```python
from build123d import *

# Parameters (mm, degrees)
SKETCH1_W           = 90
SKETCH1_H           = 90
BOSS_EXTRUDE1_DEPTH = 11.45
SKETCH2_R           = 41
BOSS_EXTRUDE2_DEPTH = 52.45
SKETCH3_R           = 29.05
BOSS_EXTRUDE3_DEPTH = 19
SKETCH4_R           = 32.5
BOSS_EXTRUDE4_DEPTH = 12
SKETCH5_R           = 28
BOSS_EXTRUDE5_DEPTH = 12
SKETCH6_R           = 2.5
CUT_EXTRUDE1_DEPTH  = 115.720105038


with BuildPart() as part:
    # Sketch1 → Boss-Extrude1 (new body)
    with BuildSketch(Plane(origin=(0, 0, 0), x_dir=(1, 0, 0), z_dir=(0, 1, 0))):
        Rectangle(SKETCH1_W, SKETCH1_H)
    extrude(amount=BOSS_EXTRUDE1_DEPTH)

    # Sketch2 → Boss-Extrude2 (add)
    with BuildSketch(Plane(origin=(0, 11.45, 0), x_dir=(1, 0, 0), z_dir=(0, 1, 0))):
        with Locations(Location((0, 0, 0), (0, 0, 270))):
            Circle(SKETCH2_R)
    extrude(amount=BOSS_EXTRUDE2_DEPTH)

    # Sketch3 → Boss-Extrude3 (add)
    with BuildSketch(Plane(origin=(0, 63.9, 0), x_dir=(1, 0, 0), z_dir=(0, 1, 0))):
        with Locations(Location((0, 0, 0), (0, 0, 270))):
            Circle(SKETCH3_R)
    extrude(amount=BOSS_EXTRUDE3_DEPTH)

    # Sketch4 → Boss-Extrude4 (add)
    with BuildSketch(Plane(origin=(0, 82.9, 0), x_dir=(1, 0, 0), z_dir=(0, 1, 0))):
        with Locations(Location((0, 0, 0), (0, 0, 270))):
            Circle(SKETCH4_R)
    extrude(amount=BOSS_EXTRUDE4_DEPTH)

    # Sketch5 → Boss-Extrude5 (add)
    with BuildSketch(Plane(origin=(0, 94.9, 0), x_dir=(1, 0, 0), z_dir=(0, 1, 0))):
        with Locations(Location((0, 0, 0), (0, 0, 270))):
            Circle(SKETCH5_R)
    extrude(amount=BOSS_EXTRUDE5_DEPTH)

    # Sketch6 → Cut-Extrude1 (cut, through all)
    with BuildSketch(Plane(origin=(0, 11.45, 0), x_dir=(1, 0, 0), z_dir=(0, 1, 0))):
        with Locations(Location((-35, 36.75, 0), (0, 0, 270))):
            Circle(SKETCH6_R)
        with Locations(Location((35, 36.75, 0), (0, 0, 270))):
            Circle(SKETCH6_R)
        with Locations(Location((35, -36.75, 0), (0, 0, 270))):
            Circle(SKETCH6_R)
        with Locations(Location((-35, -36.75, 0), (0, 0, 270))):
            Circle(SKETCH6_R)
    extrude(amount=-CUT_EXTRUDE1_DEPTH, mode=Mode.SUBTRACT)


solid = part.part
```
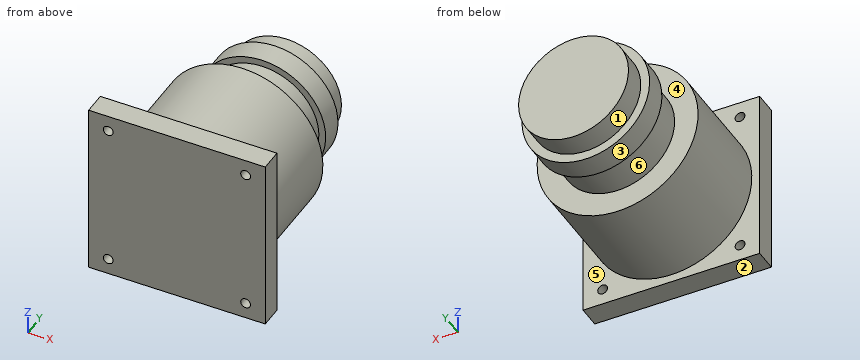
CAD build for the part. Positions are in the model's coordinates, mm. Face numbers are marked on the shaded views. A direction names the side the tool comes from. Round coordinates to 2 decimals unless told otherwise and drop trailing zeros. Write each loop counter-clockwise with the first axis right and the second up, starting at its lowest first coordinate (ties: lowest second). Pieces come first, ordered by that corner, then holes.
Item 1: Band-saw the part on B-B on x = 35. Write the cut outline in (y, z).
Filled in:
outline: (0, -45) - (11.45, -45) - (11.45, -39.25) - (0, -39.25) - close; (0, -34.25) - (11.45, -34.25) - (11.45, -21.35) - (63.9, -21.35) - (63.9, 21.35) - (11.45, 21.35) - (11.45, 34.25) - (0, 34.25) - close; (0, 39.25) - (11.45, 39.25) - (11.45, 45) - (0, 45) - close
Item 2: Drop flat-ended pins along their axis: pin 1 Ø1.5 at (y, z) = (53.5, 36) entering from -X; pin 2 Ø6.5 at (x, z) = (-35, -36.75) entering from +Y; pin 3 Ø1 at (x, y) = (-21, 53) entering from -Z; pin 4 Ø4 at (x, z) = (35, -36.75) entering from +Y. Give the stop position or say it passes through.
Filled in:
pin 1: stops at x = -20.94
pin 2: stops at y = 11.45
pin 3: stops at z = -35.51
pin 4: passes through
Item 3: Mould opens along Y. For the marked faces 3, 4, 5 and 6 say: released by +Y, released by -Y, zero draft, split by the parting line, or undercut.
Filled in:
face 3: zero draft
face 4: undercut
face 5: released by +Y
face 6: undercut
Item 4: Tool access for the marked faces 1 and 2: list every direction of +Z, -Z, +X, -X, +Y, -Y with a clear straight run to the whole face (end or side of a thin tool).
Filled in:
face 1: +Y
face 2: -Z, +X, -X, +Y, -Y
Item 5: Band-saw the part on C-C on x = 0. Write the cut outline in (y, z), then the cut area to 3 significant figures.
Filled in:
outline: (0, -45) - (11.45, -45) - (11.45, -41) - (63.9, -41) - (63.9, -29.05) - (82.9, -29.05) - (82.9, -32.5) - (94.9, -32.5) - (94.9, -28) - (106.9, -28) - (106.9, 28) - (94.9, 28) - (94.9, 32.5) - (82.9, 32.5) - (82.9, 29.05) - (63.9, 29.05) - (63.9, 41) - (11.45, 41) - (11.45, 45) - (0, 45) - close
area: 7,890 mm2
Item 6: Band-saw the part on D-D on z = 0. Write the cut outline in (x, y).
Filled in:
outline: (-45, 0) - (45, 0) - (45, 11.45) - (41, 11.45) - (41, 63.9) - (29.05, 63.9) - (29.05, 82.9) - (32.5, 82.9) - (32.5, 94.9) - (28, 94.9) - (28, 106.9) - (-28, 106.9) - (-28, 94.9) - (-32.5, 94.9) - (-32.5, 82.9) - (-29.05, 82.9) - (-29.05, 63.9) - (-41, 63.9) - (-41, 11.45) - (-45, 11.45) - close
Item 7: Band-saw the part on A-A on z = -31. Write the cut outline in (x, y).
Filled in:
outline: (-45, 0) - (45, 0) - (45, 11.45) - (26.83, 11.45) - (26.83, 63.9) - (-26.83, 63.9) - (-26.83, 11.45) - (-45, 11.45) - close; (-9.76, 82.9) - (9.76, 82.9) - (9.76, 94.9) - (-9.76, 94.9) - close
Item 8: Drill centre lines: L1, parallel to X at y = 8.25, z = -36.75; L2, parallel to Y at x = 14.5, z = 29; L3, parallel to Y at x = 19.5, z = 41.5. Where is each one in solid material? Low to high.
Filled in:
L1: x = -45 to -37.5, -32.5 to 32.5, 37.5 to 45
L2: y = 0 to 63.9, 82.9 to 94.9
L3: y = 0 to 11.45
